from build123d import *

# Parameters (mm, degrees)
F1_DEPTH = 25


with BuildPart() as f1:
    # F0 (on Front) → F1 (new body)
    with BuildSketch(Plane.XZ):
        with BuildLine():
            Line((-56.300399, -19.121413), (-42.300399, -19.121413))
            Line((-42.300399, -19.121413), (-42.300399, -24.923176))
            Line((-42.300399, -24.923176), (0, -31.121413))
            Line((0, -31.121413), (0, -39.621413))
            ThreePointArc((0, -39.621413), (0.43934, -40.682073), (1.5, -41.121413))
            Line((1.5, -41.121413), (11, -41.121413))
            ThreePointArc((11, -41.121413), (13.12132, -40.242733), (14, -38.121413))
            Line((14, -38.121413), (14, -19.121413))
            Line((14, -19.121413), (14, 31.878587))
            ThreePointArc((14, 31.878587), (13.12132, 33.999907), (11, 34.878587))
            Line((11, 34.878587), (1.5, 34.878587))
            ThreePointArc((1.5, 34.878587), (0.43934, 34.439247), (0, 33.378587))
            Line((0, 33.378587), (0, 24.878587))
            Line((0, 24.878587), (-42.300399, 19.300512))
            Line((-42.300399, 19.300512), (-42.300399, 12.878587))
            Line((-42.300399, 12.878587), (-56.300399, 12.878587))
            Line((-56.300399, 12.878587), (-56.300399, 17.454358))
            Line((-56.300399, 17.454358), (-89.696104, 13.050529))
            ThreePointArc((-89.696104, 13.050529), (-90.627865, 12.552303), (-91, 11.563403))
            Line((-91, 11.563403), (-91, -16.491046))
            ThreePointArc((-91, -16.491046), (-90.634946, -17.471809), (-89.717471, -17.975198))
            Line((-89.717471, -17.975198), (-56.300399, -22.871769))
            Line((-56.300399, -22.871769), (-56.300399, -19.121413))
        make_face()
    extrude(amount=F1_DEPTH)


solid = f1.part
Geometry: final body of the model. Coordinates: model frame, mm. A direction names the side the tool comes from. Round coordinates to 2 decimals unless told otherwise and drop trailing zeros. Loops run counter-clockwise (first coordinate to the right, second up) from the corner with the lowest first, then second, coordinate; pieces in that order, holes last.
Q1. Access query for faces 5 (the flat face through (0, -12, 29)), 6 (the flat face through (-21.45, -12.32, -27.98)), 7 (the flat face through (-49, -12, 12.879)), 8 (the flat face through (6, -12, 34.879)), 9 (the flat face through (-42.3, -12, -22)). Directions: +Z, -Z, +X, -X, +Y, -Y. A direction counts if a zero-diameter tool reaches every point of the face in a straight line with its end or side. Return the directions, or none.
Q2. Section C-C on x = -43.5. Return loops of the section in (y, z), plus the area to 3 significant figures.
Q3. Section A-A on z = 14.5. Return loops of the section in (x, y), plus the area to 3 significant figures.
Q4. Section B-B on y = -22.5. Return loops of the section in (x, z).
Q5. Pull-direction query (X, two-part tool) for faces 1 (the flat face through (-56.3, -12, 15)), 2 (the flat face through (-73.24, -12.32, -20.39)), 3 (the cylindrical face through (13.14, -12.32, 33.98)), 4 (the flat face through (-28, -25, -3)); classes: released by +X, released by -X, zero draft, split by the parting line, or undercut.
Q6. Material intervals for L1, parallel to X at y = -16.75, z = 31.5; L2, parallel to Z at x = -52, y = -15.5; L3, parallel to Z at x = -42, y = -9.25, sorted ascending.
Q7. Section D-D on z = -29.5. Return loops of the section in (x, y).
Q8. Pin query (flat end, axial travel): P1, Ø3, axis at x = -39.5, y = -16.5, coming from the -Z side; P2, Ø3, axis at y = -20, z = -25, coming from the -X side; P3, Ø7, axis at y = -13, z = 29, coming from the -X side. Return the tip coordinate at first contact, or that it passes through.
Evaluation:
1. face 5: +Z, -X, +Y, -Y
1. face 6: -Z, -X, +Y, -Y
1. face 7: +Z, +Y, -Y
1. face 8: +Z, +X, -X, +Y, -Y
1. face 9: -Z, +Y, -Y
2. outline: (-25, -19.12) - (0, -19.12) - (0, 12.88) - (-25, 12.88) - close
2. area: 800 mm2
3. outline: (-78.7, -25) - (-56.3, -25) - (-56.3, 0) - (-78.7, 0) - close; (-42.3, -25) - (14, -25) - (14, 0) - (-42.3, 0) - close
3. area: 1,970 mm2
4. outline: (-91, -16.49) arc R1.5 ccw to (-89.72, -17.98) - (-56.3, -22.87) - (-56.3, -19.12) - (-42.3, -19.12) - (-42.3, -24.92) - (0, -31.12) - (0, -39.62) arc R1.5 ccw to (1.5, -41.12) - (11, -41.12) arc R3 ccw to (14, -38.12) - (14, 31.88) arc R3 ccw to (11, 34.88) - (1.5, 34.88) arc R1.5 ccw to (0, 33.38) - (0, 24.88) - (-42.3, 19.3) - (-42.3, 12.88) - (-56.3, 12.88) - (-56.3, 17.45) - (-89.7, 13.05) arc R1.5 ccw to (-91, 11.56) - close
5. face 1: undercut
5. face 2: released by -X
5. face 3: released by +X
5. face 4: zero draft
6. L1: x = 0 to 14
6. L2: z = -19.12 to 12.88
6. L3: z = -24.97 to 19.34
7. outline: (-11.07, -25) - (14, -25) - (14, 0) - (-11.07, 0) - close
8. P1: stops at z = -25.55
8. P2: stops at x = -42.3
8. P3: stops at x = 0
